The model under review builds one solid part; all positions refer to its coordinate system, in mm. Face numbers are marked on the shaded views. Coordinates: 2 decimals unless noted, no trailing zeros. Write each loop counter-clockwise with the first axis right and the second up, starting at its lowest first coordinate (ties: lowest second). Pieces come first, ordered by that corner, then holes. Notation, with made-up numbers: (62, -23) -> (99, -23) arc R32 cw to (99, 16) -> close; hole circle Ø4 at (-35, 6). An arc over 180 degrees is marked (long way). Put each result on its own line as item: value. Start each with the question number.
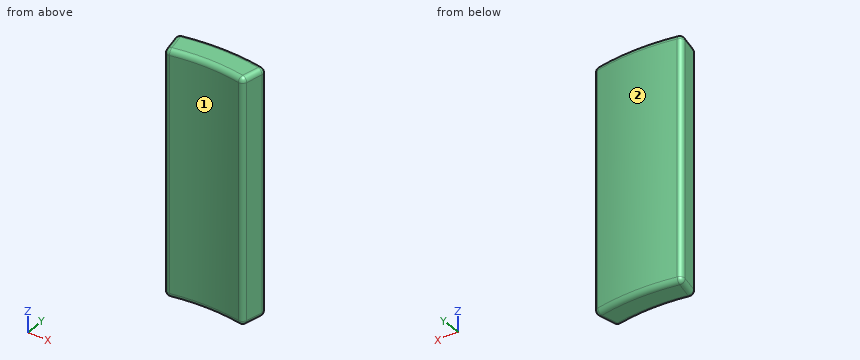
from build123d import *

# Parameters (mm, degrees)
BOSS_EXTRUDE2_DEPTH = 10
FILLET1_R           = 0.4


with BuildPart() as part:
    # Sketch4 → Boss-Extrude2 (new, symmetric)
    with BuildSketch(Plane.XY):
        with BuildLine():
            Line((-3.680036927, 0.713212533), (-3.222631208, -1.438712189))
            ThreePointArc((-3.222631208, -1.438712189), (0, -1.1), (3.222631208, -1.438712189))
            Line((3.222631208, -1.438712189), (3.680036927, 0.713212533))
            ThreePointArc((3.680036927, 0.713212533), (0, 1.1), (-3.680036927, 0.713212533))
        make_face()
    extrude(amount=BOSS_EXTRUDE2_DEPTH, both=True)

    # Fillet1
    fillet1_edges = [part.edges().sort_by_distance(p)[0] for p in [
        (0, 1.1, 10),
        (-3.451334068, -0.362749828, 10),
        (0, -1.1, 10),
        (-3.451334068, -0.362749828, -10),
        (0, 1.1, -10),
        (3.451334068, -0.362749828, -10),
        (0, -1.1, -10),
        (-3.222631208, -1.438712189, 0),
        (-3.680036927, 0.713212533, 0),
        (3.680036927, 0.713212533, 0),
        (3.222631208, -1.438712189, 0),
        (3.451334068, -0.362749828, 10),
    ]]
    fillet(fillet1_edges, radius=FILLET1_R)


solid = part.part
1. Consider section A-A on z = 5.25. State the section outline as (x, y) points.
2. Wall thickness on line 1 (Y direction, x = -0.25, z = 8.25); line 2 (Z direction, x = 0.25, y = -0.8); line 3 (Y direction, x = 3, z = -4): over which ranges is each line inside the solid? List them lowest first. Write a range as from..to.
3. Insertion check: P1, Ø4, axis at x = -2, z = 3, coming from the +Y side. The pin has a flat end and moves straight along its axis. Give the tip position at first contact, or say it passes through.
4. The part is to be moulded in two halves that separate along X. For the marked faces 1 and 2, say which applies: released by +X, released by -X, zero draft, split by the parting line, or undercut.
Output values:
1. outline: (-3.6, 0.32) -> (-3.3, -1.05) arc R0.4 ccw to (-2.84, -1.36) arc R15.5 cw to (2.84, -1.36) arc R0.4 ccw to (3.3, -1.05) -> (3.6, 0.32) arc R0.4 ccw to (3.28, 0.79) arc R17.7 ccw to (-3.28, 0.79) arc R0.4 ccw to start
2. line 1: y = -1.1..1.1
2. line 2: z = -9.99..9.99
2. line 3: y = -1.36..0.84
3. P1: stops at y = 1.1
4. face 1: undercut
4. face 2: split by the parting line
